Design review of the part built by this model. Coordinates are the model's own, in mm. A direction names the side the tool comes from. Round coordinates to 2 decimals unless told otherwise and drop trailing zeros. Order: outer loops, then holes, each group sorted by start corner. A loop starts at its lowest first (then second) coordinate and runs counter-clockwise, first axis right, second up. Notation, with made-up numbers: M 20.25,-32 L 27.25,-32 A13 ccw 27.25,-28 Z; hole C -8.5,89 d6. An arc over 180 degrees is marked long. Use a Markdown table: item, result. Add a question column.
(1) Take a section at A-A (y = 13.5). Write out the cut boundary in (x, z).
(2) Machinability: for faces 4 (the face through (-2.537, 3.131, -28.523)), 5 (the face through (4.444, 14.818, -14.112)), 6 (the face through (-34, 3.81, -2)), which of the approach directions +Z, -Z, +X, -X, +Y, -Y give a long, thin tool a straight path to every point of the face, cutting with its end or side? Answer none if there is none.
(3) For pin 1 (10 mm diameter, centred on x = 27.5, y = 13.5, fed in from +Z); pin 2 (0.7 mm diameter, centred on x = 4, y = 1.5, fed in from +Z); pin 3 (2 mm diameter, centred on y = 17.5, z = 11.5, fed in from -X), all flat-tipped, find the tip position at first contact; note any pin that passes through.
(4) To check wall thickness, follow probe 1 along Z at (x, y) = (4, 1.75); probe 2 along X at (y, z) = (5, 0); probe 3 along Z at (x, y) = (0, 4.5). State the ranges of each line that lie inside material, in increasing order. Write a range as from..to.
(5) The part is to be moulded in two halves that separate along Z. For faces 1 (the face through (-18, 0, 20)), 2 (the face through (34, 3.81, 2)), 3 (the face through (-22.41, 11.306, -29.227)), say which applies: released by +Z, released by -Z, zero draft, split by the parting line, or undercut.
```python
from build123d import *

# Parameters (mm, degrees)
SKETCH1_R           = 36.83
BOSS_EXTRUDE1_DEPTH = 20.32
FILLET1_R           = 2.54
SKETCH2_R           = 26.67
SKETCH3_R           = 14.7955
SKETCH4_R           = 14.7955
CUT_EXTRUDE1_DEPTH  = 76.2
SKETCH18_R          = 3.175
CUT_EXTRUDE2_DEPTH  = 6.35
CUT_EXTRUDE3_DEPTH  = 6.35
CUT_EXTRUDE4_START  = 2.54
CUT_EXTRUDE4_DEPTH  = 2.54
CIRPATTERN1_COUNT   = 4


with BuildPart() as part:
    # Sketch1 → Boss-Extrude1 (new body)
    with BuildSketch(Plane(origin=(0, 0, 0), x_dir=(1, 0, 0), z_dir=(0, 1, 0))):
        with Locations(Location((0, 0, 0), (0, 0, 270))):
            Circle(SKETCH1_R)
    extrude(amount=BOSS_EXTRUDE1_DEPTH)

    # Fillet1
    fillet1_edges = [part.edges().sort_by_distance(p)[0] for p in [
        (0, 0, -36.83),
    ]]
    fillet(fillet1_edges, radius=FILLET1_R)

    # Sketch2 → Cut-Loft1 section 0
    with BuildSketch(Plane(origin=(0, 0, 0), x_dir=(1, 0, 0), z_dir=(0, 1, 0))):
        Circle(SKETCH2_R)
    # Sketch3 → Cut-Loft1 section 1
    with BuildSketch(Plane(origin=(0, 11.938, 0), x_dir=(1, 0, 0), z_dir=(0, 1, 0))):
        Circle(SKETCH3_R)
    loft(mode=Mode.SUBTRACT)

    # Sketch4 → Cut-Extrude1 (cut)
    with BuildSketch(Plane.XZ.offset(-11.938)):
        with Locations(Location((0, 0, 0), (0, 0, 270))):
            Circle(SKETCH4_R)
    extrude(amount=-CUT_EXTRUDE1_DEPTH, mode=Mode.SUBTRACT)

    # Sketch17 → Cut-Revolve1 (revolve, cut)
    with BuildSketch(Plane(origin=(0, 0, 0), x_dir=(0, 0, -1), z_dir=(1, 0, 0))):
        with BuildLine():
            Line((36.83, 20.32), (14.7955, 20.32))
            Line((14.7955, 20.32), (14.7955, 17.78))
            ThreePointArc((14.7955, 17.78), (26.041766832, 17.063278986), (36.83, 20.32))
        make_face()
    revolve(axis=Axis((0, 0, 0), (0, 1, 0)), mode=Mode.SUBTRACT)

    # Sketch18 → Cut-Extrude2 (cut)
    with BuildSketch(Plane.XZ):
        with Locations(Location((0, 30.431156816, 0), (0, 0, 270))):
            Circle(SKETCH18_R)
        with Locations(Location((-30.431156816, 0, 0), (0, 0, 270))):
            Circle(SKETCH18_R)
        with Locations(Location((0, -30.431156816, 0), (0, 0, 270))):
            Circle(SKETCH18_R)
        with Locations(Location((30.431156816, 0, 0), (0, 0, 270))):
            Circle(SKETCH18_R)
    extrude(amount=-CUT_EXTRUDE2_DEPTH, mode=Mode.SUBTRACT)

    # Sketch19 → Cut-Extrude3 (cut)
    with BuildSketch(Plane.XZ):
        with BuildLine():
            Line((4.259709497, -31.701156816), (2.909935566, -31.701156816))
            ThreePointArc((2.909935566, -31.701156816), (3.175, -30.431156816), (2.909935566, -29.161156816))
            Line((2.909935566, -29.161156816), (4.259709497, -29.161156816))
            ThreePointArc((4.259709497, -29.161156816), (4.445, -30.431156816), (4.259709497, -31.701156816))
        make_face()
    cut_extrude3 = extrude(amount=-CUT_EXTRUDE3_DEPTH, mode=Mode.SUBTRACT)

    # Sketch20 → Cut-Extrude4 (cut)
    with BuildSketch(Plane.XZ.offset(-6.35).offset(CUT_EXTRUDE4_START)):
        with BuildLine():
            Line((-1.27, -34.690866313), (-1.27, -33.341092382))
            ThreePointArc((-1.27, -33.341092382), (1.15960956, -33.3868176), (2.909935566, -31.701156816))
            Line((2.909935566, -31.701156816), (4.259709497, -31.701156816))
            ThreePointArc((4.259709497, -31.701156816), (2.114043859, -34.341251899), (-1.27, -34.690866313))
        make_face()
    cut_extrude4 = extrude(amount=-CUT_EXTRUDE4_DEPTH, mode=Mode.SUBTRACT)

    # CirPattern1: Cut-Extrude3, Cut-Extrude4 ×4 about axis
    cirpattern1_axis = Axis((0, 0, 0), (0, 1, 0))
    add([cut_extrude3.rotate(cirpattern1_axis, i * 360 / CIRPATTERN1_COUNT) for i in range(1, CIRPATTERN1_COUNT)], mode=Mode.SUBTRACT)
    add([cut_extrude4.rotate(cirpattern1_axis, i * 360 / CIRPATTERN1_COUNT) for i in range(1, CIRPATTERN1_COUNT)], mode=Mode.SUBTRACT)


solid = part.part
```
Verdict:
| question | item | result |
|---|---|---|
| 1 | outline | C 0,0 d73.66; hole C 0,0 d29.59 |
| 2 | face 4 | -Y |
| 2 | face 5 | +Y, -Y |
| 2 | face 6 | none |
| 3 | pin 1 | stops at z = 29.16 |
| 3 | pin 2 | stops at z = 36.52 |
| 3 | pin 3 | stops at x = -35.3 |
| 4 | probe 1 | z = -36.49..-31.7, -29.16..-24.61, 24.61..36.49 |
| 4 | probe 2 | x = -36.83..-34.88, -27.26..-21.7, 21.7..27.26, 34.88..36.83 |
| 4 | probe 3 | z = -36.83..-34.88, -27.26..-22.19, 22.19..27.26, 34.88..36.83 |
| 5 | face 1 | zero draft |
| 5 | face 2 | undercut |
| 5 | face 3 | split by the parting line |
